Could you check a few things on this model? Use its own coordinates, in mm. A direction names the side the tool comes from. Give positions to 0.01 mm unless a question says otherwise; leave off trailing zeros. Loops run counter-clockwise (first coordinate to the right, second up) from the corner with the lowest first, then second, coordinate; pieces in that order, holes last. Notation, with made-up numbers: (51, -3) - (64, -3) arc R19 cw to (64, 19) - close; hole circle Ø2 at (2.25, 50.5). An arc over 180 degrees is marked (long way). Use CSV: the item, a comma, the result in double quotes.
from build123d import *

# Parameters (mm, degrees)
F1_DEPTH = 40
F2_W     = 5.6
F2_H     = 13.2
F3_DEPTH = 10


with BuildPart() as f1:
    # F0 (on Front) → F1 (new body, symmetric)
    with BuildSketch(Plane.XZ):
        with BuildLine():
            Line((-9.5, -10.7), (9.5, -10.7))
            ThreePointArc((9.5, -10.7), (14.240517, -9.592713), (18, -6.5))
            Line((18, -6.5), (18, 6.5))
            ThreePointArc((18, 6.5), (14.240517, 9.592713), (9.5, 10.7))
            Line((9.5, 10.7), (-9.5, 10.7))
            ThreePointArc((-9.5, 10.7), (-14.240517, 9.592713), (-18, 6.5))
            Line((-18, 6.5), (-18, -6.5))
            ThreePointArc((-18, -6.5), (-14.240517, -9.592713), (-9.5, -10.7))
        make_face()
    extrude(amount=F1_DEPTH, both=True)

    # F2 (on face) → F3 (cut)
    with BuildSketch(Plane.XZ.offset(40)):
        with Locations((10.8, 0)):
            Rectangle(F2_W, F2_H)
    extrude(amount=-F3_DEPTH, mode=Mode.SUBTRACT)


solid = f1.part
1) Which directions (+Z, -Z, +X, -X, +Y, -Y) give clear straight access to the entire face, cutting with the end or side of a thin tool? Please do faces 1 (the flat face through (11, -35, 6.6)), 2 (the cylindrical face through (-14.179, -0.56, 9.623)).
Answer below:
face 1,"-Y"
face 2,"+Z, -X, +Y, -Y"
2) Suppose I cut it at B-B (z = 1). Please give me the cut outline in (x, y), plus the area to 3 significant figures.
Answer below:
outline,"(-18, -40) - (8, -40) - (8, -30) - (13.6, -30) - (13.6, -40) - (18, -40) - (18, 40) - (-18, 40) - close"
area,"2,820 mm2"
3) I need wall thicknesses on line 1 along X through (y, z) = (-37, 4.5); line 2 along Y through (x, z) = (11.5, 2); line 3 along X through (y, z) = (1.5, 8.25). Which ranges of each line are inside material? Lowest first, please.
Answer below:
line 1,"x = -18 to 8, 13.6 to 18"
line 2,"y = -30 to 40"
line 3,"x = -16.31 to 16.31"
4) Suppose I cut it at C-C (x = -11.5). Please give me the cut outline in (y, z).
Answer below:
outline,"(-40, -10.51) - (40, -10.51) - (40, 10.51) - (-40, 10.51) - close"
5) I'm going to push flat-ended pins straight in: P1, Ø6, axis at y = 10.5, z = 8, coming from the +X side; P2, Ø4.5, axis at x = 12, y = -35.5, coming from the -Z side. Where does each tip first touch, or does it pass through?
Answer below:
P1,"stops at x = 18"
P2,"stops at z = -10.7"
6) Suppose I cut it at A-A (y = 34). Please give me the cut outline in (x, z).
Answer below:
outline,"(-18, -6.5) arc R10.7 ccw to (-9.5, -10.7) - (9.5, -10.7) arc R10.7 ccw to (18, -6.5) - (18, 6.5) arc R10.7 ccw to (9.5, 10.7) - (-9.5, 10.7) arc R10.7 ccw to (-18, 6.5) - close"
7) We'd pull the mould along Z, two halves only. Please class faces 3 (the flat face through (11, -30, 0)), 4 (the cylindrical face through (-14.302, -0.56, -9.562)), 5 (the flat face through (0, -40, 0)): +Z half, -Z half, draft (parallel to the pull), parting line (faces both ways), or undercut.
Answer below:
face 3,"undercut"
face 4,"-Z half"
face 5,"draft"
